Design review of the part shown in the three views and the two pictorial views. Dimensions are in mm from the part's minimum x, y and z. A direction names the side the tool comes from. Give positions to 0.01 mm unless a question says otherwise; leave off trailing zeros. Loops run counter-clockwise (first coordinate to the right, second up) from the corner with the lowest first, then second, coordinate; pieces in that order, holes last.
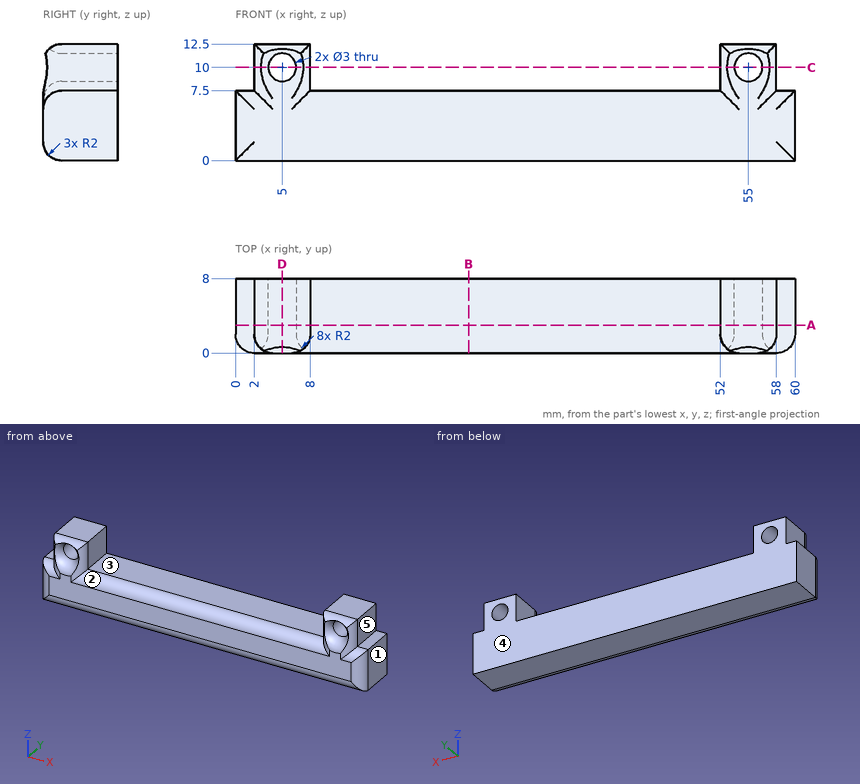
Q1. Take a section at A-A (y = 3). Give the boundary of the cut face in (x, z), plus the area to 3 significant figures.
Results:
outline: (0, 0) - (60, 0) - (60, 7.5) - (58, 7.5) - (58, 12.5) - (52, 12.5) - (52, 7.5) - (8, 7.5) - (8, 12.5) - (2, 12.5) - (2, 7.5) - (0, 7.5) - close; hole circle Ø3 at (5, 10); hole circle Ø3 at (55, 10)
area: 496 mm2
Q2. Insertion check: pin 1 (1.5 mm diameter, centred on y = 5.5, z = 10.5, fed in from +X); pin 2 (1 mm diameter, centred on x = 27.5, y = 1.5, fed in from +Z); pin 3 (5 mm diameter, centred on x = 5, z = 10, fed in from -Y). Each pin has a flat end and moves straight along its axis. Give the tip position at first contact, or say it passes through.
Results:
pin 1: stops at x = 58
pin 2: stops at z = 7.5
pin 3: stops at y = 0.27
Q3. Wall thickness on line 1 (Z direction, x = 5, y = 4.8); line 2 (X direction, y = 3, z = 11.25); line 3 (X direction, y = 7.25, z = 11): over which ranges is each line inside the solid? List them lowest first.
Results:
line 1: z = 0 to 8.5, 11.5 to 12.5
line 2: x = 2 to 4.17, 5.83 to 8, 52 to 54.17, 55.83 to 58
line 3: x = 2 to 3.88, 6.12 to 8, 52 to 53.88, 56.12 to 58
Q4. Take a section at B-B (x = 25). Give the boundary of the cut face in (y, z), plus the area to 3 significant figures.
Results:
outline: (0, 2) arc R2 ccw to (2, 0) - (8, 0) - (8, 7.5) - (2, 7.5) arc R2 ccw to (0, 5.5) - close
area: 58.3 mm2
Q5. Take a section at D-D (x = 5). Give the boundary of the cut face in (y, z).
Results:
outline: (0, 2) arc R2 ccw to (2, 0) - (8, 0) - (8, 8.5) - (2, 8.5) arc R2 ccw to (0, 6.5) - close; (0.68, 12) arc R2 ccw to (2, 11.5) - (8, 11.5) - (8, 12.5) - (2, 12.5) arc R2 ccw to start
Q6. Take a section at C-C (z = 10). Give the boundary of the cut face in (x, y), plus the area to 3 significant figures.
Results:
outline: (2, 2) arc R2 ccw to (2.75, 0.44) arc R2 ccw to (3.5, 2) - (3.5, 8) - (2, 8) - close; (6.5, 2) arc R2 ccw to (7.25, 0.44) arc R2 ccw to (8, 2) - (8, 8) - (6.5, 8) - close; (52, 2) arc R2 ccw to (52.75, 0.44) arc R2 ccw to (53.5, 2) - (53.5, 8) - (52, 8) - close; (56.5, 2) arc R2 ccw to (57.25, 0.44) arc R2 ccw to (58, 2) - (58, 8) - (56.5, 8) - close
area: 42.5 mm2
Q7. Tool access review of the marked faces 1, 2, 3, 4 and 5: name each direction out of +Z, -Z, +X, -X, +Y, -Y from which nothing blocks a thin tool from reaching the whole face with its end or side.
Results:
face 1: +Z, -Z, +X, +Y, -Y
face 2: +Z, -Y
face 3: +Z, +Y, -Y
face 4: +Z, -Z, +X, -X, +Y
face 5: +Z, +X, +Y, -Y
